from build123d import *

# Parameters (mm, degrees)
F0_R     = 4.25
F1_DEPTH = 25
F2_R     = 12.507492
F3_R     = 5


with BuildPart() as f1:
    # F0 (on Top) → F1 (new body)
    with BuildSketch(Plane.XY):
        with BuildLine():
            Line((0, 93.520519), (-99.141695, -54.804042))
            Line((-99.141695, -54.804042), (-39.790552, -54.804042))
            ThreePointArc((-39.790552, -54.804042), (-28.136169, -26.667873), (0, -15.01349))
            ThreePointArc((0, -15.01349), (28.136169, -26.667873), (39.790552, -54.804042))
            Line((39.790552, -54.804042), (99.141695, -54.804042))
            Line((99.141695, -54.804042), (0, 93.520519))
        make_face()
        with Locations((-67.721896, -44.267751)):
            Circle(F0_R, mode=Mode.SUBTRACT)
        with Locations((67.721896, -44.267751)):
            Circle(F0_R, mode=Mode.SUBTRACT)
        with Locations((0, 72.195958)):
            Circle(F0_R, mode=Mode.SUBTRACT)
    extrude(amount=F1_DEPTH)

    # F2
    f2_edges = [f1.edges().sort_by_distance(p)[0] for p in [
        (0, 93.520519, 12.5),
    ]]
    fillet(f2_edges, radius=F2_R)

    # F3
    f3_edges = [f1.edges().sort_by_distance(p)[0] for p in [
        (-39.790552, -54.804042, 12.5),
        (39.790552, -54.804042, 12.5),
        (99.141695, -54.804042, 12.5),
        (-99.141695, -54.804042, 12.5),
    ]]
    fillet(f3_edges, radius=F3_R)


solid = f1.part
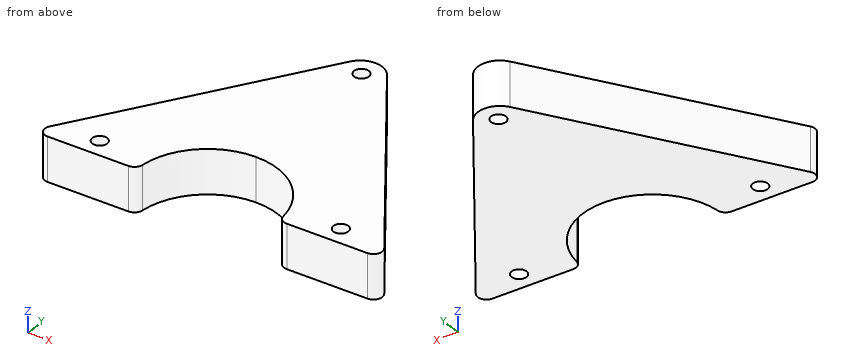
Part model, mm, in its own coordinate system. Round coordinates to 2 decimals unless told otherwise and drop trailing zeros. Write each loop counter-clockwise with the first axis right and the second up, starting at its lowest first coordinate (ties: lowest second). Pieces come first, ordered by that corner, then holes. Notation, with made-up numbers: M 30,77.25 L 74,77.25 A26 ccw 74,115.25 Z; hole C 6.25,29 d7. An arc over 180 degrees is marked long. Return JSON: item names as keys, results as strings. Group by question number.
(1) Pin check, flat tips, straight feed: pin 1 Ø6 at (y, z) = (-5, 13) entering from +X; pin 2 Ø1.5 at (x, z) = (19.5, 19.5) entering from -Y; pin 3 Ø12 at (y, z) = (28.5, 13) entering from +X; pin 4 Ø13.5 at (x, y) = (-67.72, -44.27) entering from -Z. Stop position of each tip, or through.
(2) Drill centre lines: probe 1 along X at (y, z) = (-43, 3); probe 2 along Y at (x, z) = (69.5, 21.5); probe 3 along X at (y, z) = (-23, 1). Where is each one in solid material? Low to high.
(3) Saw through at B-B on x = -49. Write the cut outline in (y, z).
(4) Saw through at C-C on y = 27.5. Write the cut outline in (x, z).
(5) Saw through at A-A on z = 16. Write the cut outline in (x, y), then the cut area to 3 significant figures.
Returned:
{
 "1": {"pin 1": "x = 67.86", "pin 2": "y = -20.55", "pin 3": "x = 47.47", "pin 4": "z = 0"},
 "2": {"probe 1": "-91.25 to -71.78, -63.67 to -38, 38 to 63.67, 71.78 to 91.25", "probe 2": "-54.8 to -48.13, -40.41 to -10.46", "probe 3": "-77.88 to -23.91, 23.91 to 77.88"},
 "3": {"outline": "M -54.8,0 L 20.21,0 L 20.21,25 L -54.8,25 Z"},
 "4": {"outline": "M -44.13,0 L 44.13,0 L 44.13,25 L -44.13,25 Z"},
 "5": {"outline": "M -93.94,-47.03 A5 ccw -89.79,-54.8 L -44.51,-54.8 A5 ccw -39.54,-50.36 A39.79 cw 39.54,-50.36 A5 ccw 44.51,-54.8 L 89.79,-54.8 A5 ccw 93.94,-47.03 L 10.4,77.96 A12.51 ccw -10.4,77.96 Z; hole C -67.72,-44.27 d8.5; hole C 0,72.2 d8.5; hole C 67.72,-44.27 d8.5", "area": "11,900 mm²"}
}
